Part model, mm, in its own coordinate system. Face numbers are marked on the shaded views. A direction names the side the tool comes from. Coordinates: 2 decimals unless noted, no trailing zeros. Order: outer loops, then holes, each group sorted by start corner. A loop starts at its lowest first (then second) coordinate and runs counter-clockwise, first axis right, second up.
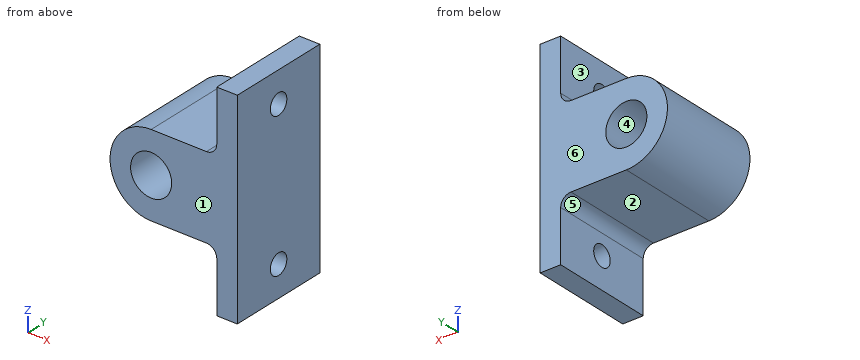
from build123d import *

# Parameters (mm, degrees)
SKETCH1_R           = 4
BOSS_EXTRUDE1_DEPTH = 20
SKETCH2_R           = 2
CUT_EXTRUDE1_DEPTH  = 20
FILLET1_R           = 2


with BuildPart() as part:
    # Sketch1 → Boss-Extrude1 (new body)
    with BuildSketch(Plane(origin=(0, 0, 0), x_dir=(1, 0, 0), z_dir=(0, 1, 0))):
        with BuildLine():
            Line((-14.775, 8), (-2, 8))
            Line((-2, 8), (-2, 20))
            Line((-2, 20), (2, 20))
            Line((2, 20), (2, -20))
            Line((2, -20), (-2, -20))
            Line((-2, -20), (-2, -8))
            Line((-2, -8), (-14.775, -8))
            ThreePointArc((-14.775, -8), (-22.775, 0), (-14.775, 8))
        make_face()
        with Locations(Location((-14.775, 0, 0), (0, 0, 270))):
            Circle(SKETCH1_R, mode=Mode.SUBTRACT)
    extrude(amount=BOSS_EXTRUDE1_DEPTH)

    # Sketch2 → Cut-Extrude1 (cut)
    with BuildSketch(Plane.ZY.offset(2)):
        with Locations((-14, 10)):
            Circle(SKETCH2_R)
        with Locations((14, 10)):
            Circle(SKETCH2_R)
    extrude(amount=-CUT_EXTRUDE1_DEPTH, mode=Mode.SUBTRACT)

    # Fillet1
    fillet1_edges = [part.edges().sort_by_distance(p)[0] for p in [
        (-2, 10, 8),
        (-2, 10, -8),
    ]]
    fillet(fillet1_edges, radius=FILLET1_R)


solid = part.part
Q1. Pin check, flat tips, straight feed: pin 1 Ø5 at (x, y) = (-7, 16.5) entering from +Z; pin 2 Ø8 at (y, z) = (6, 5) entering from -X; pin 3 Ø5 at (y, z) = (7, -15.5) entering from -X. Stop position of each tip, or through.
Results list:
pin 1: stops at z = 8
pin 2: stops at x = -22.71
pin 3: stops at x = -2
Q2. Which spindle directions (+Z, -Z, +X, -X, +Y, -Y) get a long thin tool onto all of the face, cutting with end or side? Do the marked faces 1, 2 and 3. Say none if no direction does.
Results list:
face 1: +Z, -Z, +X, -X, -Y
face 2: -Z, -X, +Y, -Y
face 3: +Z, -X, +Y, -Y
Q3. Cut at D-D on y = 3.75. Write the cut outline in (x, z) (3 decimals).
Results list:
outline: (-14.775, -8) - (-4, -8) arc R2 cw to (-2, -10) - (-2, -20) - (2, -20) - (2, 20) - (-2, 20) - (-2, 10) arc R2 cw to (-4, 8) - (-14.775, 8) arc R8 ccw to start; hole circle Ø8 at (-14.775, 0)
Q4. Cut at B-B on z = 0. Write the cut outline in (x, y) (3 decimals), and give its area (4 significant figures).
Results list:
outline: (-22.775, 0) - (-18.775, 0) - (-18.775, 20) - (-22.775, 20) - close; (-10.775, 0) - (2, 0) - (2, 20) - (-10.775, 20) - close
area: 335.5 mm2
Q5. Cut at C-C on x = -17. Write the cut outline in (y, z), and give its area (3 significant figures).
Results list:
outline: (0, -7.68) - (20, -7.68) - (20, -3.32) - (0, -3.32) - close; (0, 3.32) - (20, 3.32) - (20, 7.68) - (0, 7.68) - close
area: 174 mm2
Q6. Mould opens along Z. For the marked faces 4, 5 and 6 say: pulls with the +Z half, pulls with the -Z half, needs draft (parallel to the pull), parting line crosses it, or undercut.
Results list:
face 4: undercut
face 5: pulls with the -Z half
face 6: needs draft
Q7. Cut at A-A on y = 10. Write the cut outline in (x, z) (3 decimals).
Results list:
outline: (-14.775, -8) - (-4, -8) arc R2 cw to (-2, -10) - (-2, -12) - (2, -12) - (2, 12) - (-2, 12) - (-2, 10) arc R2 cw to (-4, 8) - (-14.775, 8) arc R8 ccw to start; (-2, -20) - (2, -20) - (2, -16) - (-2, -16) - close; (-2, 16) - (2, 16) - (2, 20) - (-2, 20) - close; hole circle Ø8 at (-14.775, 0)
Q8. Wall check: line 1 along Y through (x, z) = (0.8, 14); line 2 along Z through (x, y) = (-0.25, 10.75); line 3 along X through (y, z) = (13, 0) (3 decimals). Give the ranges that are in metal, low to high.
Results list:
line 1: y = 0 to 8, 12 to 20
line 2: z = -20 to -15.85, -12.15 to 12.15, 15.85 to 20
line 3: x = -22.775 to -18.775, -10.775 to 2
